Autodesk Inventor part; units mm, degrees
ref_plane "YZ Plane" through (0, 0, 0) normal (1, 0, 0) x (0, 1, 0)
ref_plane "XZ Plane" through (0, 0, 0) normal (0, 1, 0) x (-1, 0, 0)
ref_plane "XY Plane" through (0, 0, 0) normal (0, 0, 1) x (1, 0, 0)
sketch "Sketch1" plane through (0, 0, 0) normal (0, 0, 1) x (1, 0, 0)
  circle A0 centre (0, 0) radius 10
  circle A1 centre (0, 15) radius 5
  line L0 (0, 0) -> (0, 15)
  line L1 (-4.714, 16.6667) -> (-9.4281, 3.3333)
  line L2 (4.714, 16.6667) -> (9.4281, 3.3333)
  dimension "d0" = 20
  dimension "d1" = 10
extrude "Extrusion1" add sketch "Sketch1" along normal blind 1.6
sketch "Sketch2" plane through (0, 0, 1.6) normal (0, 0, 1) x (1, 0, 0)
  arc A0 (-9.4281, 3.3333) -> (9.4281, 3.3333) centre (0, 0) ccw
  line L0 (9.4281, 3.3333) -> (4.714, 16.6667)
  arc A1 (4.714, 16.6667) -> (-4.714, 16.6667) centre (0, 15) ccw
  line L1 (-4.714, 16.6667) -> (-9.4281, 3.3333)
hole "Hole1" at (0, 15, 1.6) direction (0, 0, -1) diameter 5 end through all
sketch "Sketch3" plane through (0, 0, 1.6) normal (0, 0, 1) x (1, 0, 0)
  circle A0 centre (0, 15) radius 2.5
  point P0 (0, 0)
properties part number "Key Fob" material "ABS Plastic"
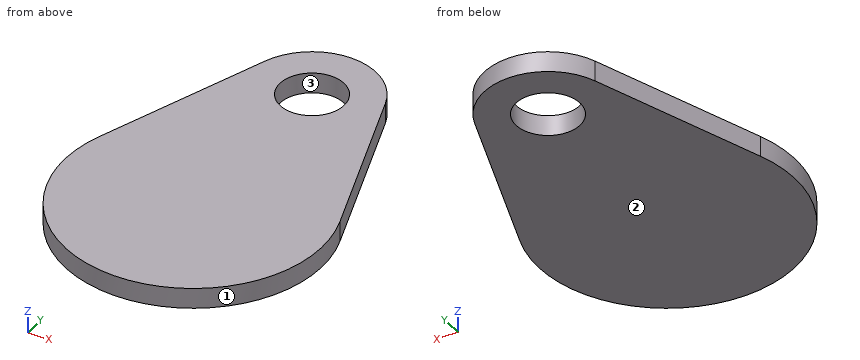
Verification items for the finished model (mm, model axes). Face numbers are marked on the shaded views. Coordinates: 2 decimals unless noted, no trailing zeros. Order: outer loops, then holes, each group sorted by start corner. A loop starts at its lowest first (then second) coordinate and runs counter-clockwise, first axis right, second up. Notation, with made-up numbers: M -28,63.25 L -7,63.25 A29 ccw -7,95.25 Z; hole C 30,-21 d10. An arc over 180 degrees is marked long. One line per item, written item: value. Start each with the question number.
Item 1: Sectioned sample at C-C (z = 1.35). Enter the section's corners in (x, y).
Item 2: Mould release check, pull along Y, two halves, no side actions. Record for the marked faces 1, 2 and 3: released by +Y, released by -Y, zero draft, split by the parting line, or undercut.
Item 3: Scan lines: probe 1 along Y at (x, z) = (0, 0.3); probe 2 along Y at (x, z) = (-0.75, 1.4); probe 3 along X at (y, z) = (15, 0.9). Record each from-to range of solid material in increasing order.
Item 4: Sectioned sample at B-B (y = 15). Enter the section's corners in (x, z), then the cut area to 3 significant figures.
Item 5: Sectioned sample at A-A (x = 0). Enter the section's corners in (y, z), then the cut area to 3 significant figures.
Item 6: Sectioned sample at D-D (y = -6). Enter the section's corners in (x, z), then the cut area to 3 significant figures.
Conclusion:
1. outline: M -9.43,3.33 A10 ccw long 9.43,3.33 L 4.71,16.67 A5 ccw -4.71,16.67 Z; hole C 0,15 d5
2. face 1: split by the parting line
2. face 2: zero draft
2. face 3: undercut
3. probe 1: y = -10 to 12.5, 17.5 to 20
3. probe 2: y = -9.97 to 12.62, 17.38 to 19.94
3. probe 3: x = -5.3 to -2.5, 2.5 to 5.3
4. outline: M -5.3,0 L -2.5,0 L -2.5,1.6 L -5.3,1.6 Z; M 2.5,0 L 5.3,0 L 5.3,1.6 L 2.5,1.6 Z
4. area: 8.97 mm^2
5. outline: M -10,0 L 12.5,0 L 12.5,1.6 L -10,1.6 Z; M 17.5,0 L 20,0 L 20,1.6 L 17.5,1.6 Z
5. area: 40.0 mm^2
6. outline: M -8,0 L 8,0 L 8,1.6 L -8,1.6 Z
6. area: 25.6 mm^2
